Could you check a few things on this drawing? It's one solid part, dimensions in mm from its lowest x, y, z. Coordinates: 2 decimals unless noted, no trailing zeros. Order: outer loops, then holes, each group sorted by start corner. A loop starts at its lowest first (then second) coordinate and runs counter-clockwise, first axis right, second up. Notation, with made-up numbers: (-20.5, -18) - (-16.5, -18) arc R19 cw to (-16.5, -8) - close; hole circle Ø11 at (21, -1.5). An arc over 180 degrees is marked (long way). Return JSON: item names as keys, results as strings. Group by question number.
1) Imagine slicing it at C-C (x = 10). Write out the boundary of the cut face in (y, z).
2) Imagine slicing it at A-A (x = 25). Write out the boundary of the cut face in (y, z), and give its area (3 significant figures).
3) If I drill on line 1 along Y through (x, z) = (40, 0.6); line 2 along Y through (x, z) = (10.5, 0.8), over which ranges is the centre line in solid material (lowest first)?
4) Imagine slicing it at B-B (z = 1.2). Write out the boundary of the cut face in (x, y).
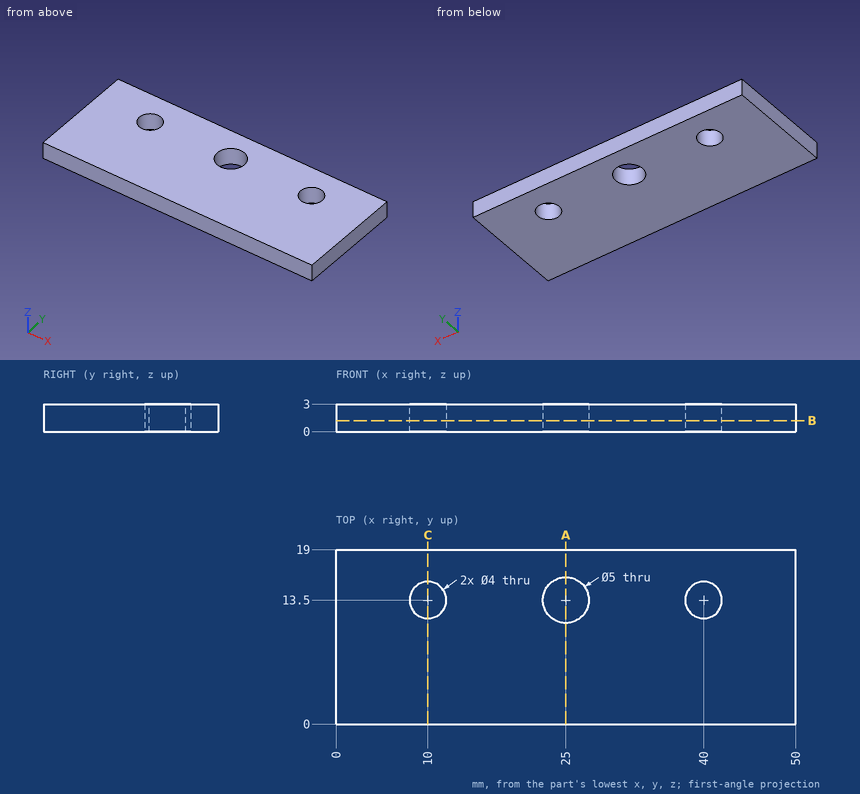
Calculated:
{
 "1": {"outline": "(0, 0) - (11.5, 0) - (11.5, 3) - (0, 3) - close; (15.5, 0) - (19, 0) - (19, 3) - (15.5, 3) - close"},
 "2": {"outline": "(0, 0) - (11, 0) - (11, 3) - (0, 3) - close; (16, 0) - (19, 0) - (19, 3) - (16, 3) - close", "area": "42.0 mm2"},
 "3": {"line 1": "0 to 11.5, 15.5 to 19", "line 2": "0 to 11.56, 15.44 to 19"},
 "4": {"outline": "(0, 0) - (50, 0) - (50, 19) - (0, 19) - close; hole circle Ø4 at (10, 13.5); hole circle Ø5 at (25, 13.5); hole circle Ø4 at (40, 13.5)"}
}
